from build123d import *

# Parameters (mm, degrees)
SKETCH1_R           = 30
BOSS_EXTRUDE1_DEPTH = 9.1
FILLET1_R           = 1.5
SKETCH2_W           = 47
SKETCH2_H           = 36.6
CUT_EXTRUDE1_DEPTH  = 4.1
SKETCH3_R           = 1.5
CUT_EXTRUDE2_DEPTH  = 43.720018867
CUT_EXTRUDE3_DEPTH  = 3
SKETCH5_R           = 1
CUT_EXTRUDE4_DEPTH  = 43.862687891


with BuildPart() as part:
    # Sketch1 → Boss-Extrude1 (new body)
    with BuildSketch(Plane(origin=(0, 0, 0), x_dir=(1, 0, 0), z_dir=(0, 1, 0))):
        with Locations(Location((0, 0, 0), (0, 0, 270))):
            Circle(SKETCH1_R)
    extrude(amount=BOSS_EXTRUDE1_DEPTH)

    # Fillet1
    fillet1_edges = [part.edges().sort_by_distance(p)[0] for p in [
        (0, 9.1, -30),
    ]]
    fillet(fillet1_edges, radius=FILLET1_R)

    # Sketch2 → Cut-Extrude1 (cut)
    with BuildSketch(Plane(origin=(0, 9.1, 0), x_dir=(1, 0, 0), z_dir=(0, 1, 0))):
        Rectangle(SKETCH2_W, SKETCH2_H)
    extrude(amount=-CUT_EXTRUDE1_DEPTH, mode=Mode.SUBTRACT)

    # Sketch3 → Cut-Extrude2 (cut, through all)
    with BuildSketch(Plane(origin=(0, 5, 0), x_dir=(1, 0, 0), z_dir=(0, 1, 0))):
        with Locations(Location((11.75, 0, 0), (0, 0, 270))):
            Circle(SKETCH3_R)
        with Locations(Location((-11.75, 0, 0), (0, 0, 90))):
            Circle(SKETCH3_R)
    extrude(amount=-CUT_EXTRUDE2_DEPTH, mode=Mode.SUBTRACT)

    # Sketch4 → Cut-Extrude3 (cut)
    with BuildSketch(Plane.XZ):
        with BuildLine():
            Line((-2.389129319, 14.428169014), (-3.73301456, 0.356514085))
            ThreePointArc((-3.73301456, 0.356514085), (-3.75, 0), (-3.73301456, -0.356514085))
            Line((-3.73301456, -0.356514085), (-2.389129319, -14.428169014))
            ThreePointArc((-2.389129319, -14.428169014), (0, -16.6), (2.389129319, -14.428169014))
            Line((2.389129319, -14.428169014), (3.73301456, -0.356514085))
            ThreePointArc((3.73301456, -0.356514085), (3.75, 0), (3.73301456, 0.356514085))
            Line((3.73301456, 0.356514085), (2.389129319, 14.428169014))
            ThreePointArc((2.389129319, 14.428169014), (0, 16.6), (-2.389129319, 14.428169014))
        make_face()
    extrude(amount=-CUT_EXTRUDE3_DEPTH, mode=Mode.SUBTRACT)

    # Sketch5 → Cut-Extrude4 (cut, through all)
    with BuildSketch(Plane.XZ.offset(-3)):
        with Locations(Location((0, 0, 0), (0, 0, 270))):
            Circle(SKETCH5_R)
    extrude(amount=-CUT_EXTRUDE4_DEPTH, mode=Mode.SUBTRACT)


solid = part.part
Model file for the job. Use its own axes, mm. A direction names the side the tool comes from. Give positions to 0.01 mm unless a question says otherwise; leave off trailing zeros. Loops run counter-clockwise (first coordinate to the right, second up) from the corner with the lowest first, then second, coordinate; pieces in that order, holes last. Notation, with made-up numbers: (20, 77.5) -> (49, 77.5) arc R11 cw to (49, 85.5) -> close; hole circle Ø7 at (-8.75, 37). An arc over 180 degrees is marked (long way). Use a Markdown table: item, result. Add a question column.
(1) Wall check: line 1 along X through (y, z) = (2.6, 0); line 2 along X through (y, z) = (3.7, 0); line 3 along Z through (x, y) = (23, 8). Give the ranges that are in metal, low to high.
(2) Tool access for faces 4 (the flat face through (23.5, 7, 0)), 5 (the cylindrical face through (0, 1.5, 16.6)), 6 (the flat face through (-25, 9.1, 0)): list every direction of +Z, -Z, +X, -X, +Y, -Y with a clear straight run to the whole face (end or side of a thin tool).
(3) Slice it at A-A on x = 0. List the corners of the cut face in (y, z), and give its area (3 significant figures).
(4) Slice it at B-B on y = 1.25. List the corners of the cut face in (x, z), and give its area (3 significant figures).
(5) Drop flat-ended pins along their axis: pin 1 Ø1.2 at (x, y) = (-1.5, 7.5) entering from -Z; pin 2 Ø1.5 at (x, z) = (-10.5, 6.5) entering from +Y; pin 3 Ø1.5 at (y, z) = (2, 9.5) entering from +X; pin 4 Ø8.5 at (x, z) = (-1.5, -4) entering from -Y. Give the stop position or say it passes through.
(6) Mould opens along X. For faces 1 (the flat face through (0, 7, -18.3)), 2 (the flat face through (-6, 0, 0)), 3 (the flat face through (2, 3, 0)) say: +X half, -X half, draft (parallel to the pull), parting line (faces both ways), or undercut.
(7) Slice it at C-C on y = 6. List the corners of the cut face in (x, z).
Filled sheet:
| question | item | result |
|---|---|---|
| 1 | line 1 | -30 to -13.25, -10.25 to -3.75, 3.75 to 10.25, 13.25 to 30 |
| 1 | line 2 | -30 to -13.25, -10.25 to -1, 1 to 10.25, 13.25 to 30 |
| 1 | line 3 | -19.18 to -18.3, 18.3 to 19.18 |
| 2 | face 4 | +Y |
| 2 | face 5 | -Y |
| 2 | face 6 | +Z, -Z, +X, -X, +Y |
| 3 | outline | (0, -30) -> (7.6, -30) arc R1.5 ccw to (9.1, -28.5) -> (9.1, -18.3) -> (5, -18.3) -> (5, -1) -> (3, -1) -> (3, -16.6) -> (0, -16.6) -> close; (0, 16.6) -> (3, 16.6) -> (3, 1) -> (5, 1) -> (5, 18.3) -> (9.1, 18.3) -> (9.1, 28.5) arc R1.5 ccw to (7.6, 30) -> (0, 30) -> close |
| 3 | area | 291 mm2 |
| 4 | outline | circle Ø60 at (0, 0); hole circle Ø3 at (-11.75, 0); hole (-3.73, -0.36) -> (-2.39, -14.43) arc R2.4 ccw to (2.39, -14.43) -> (3.73, -0.36) arc R3.75 ccw to (3.73, 0.36) -> (2.39, 14.43) arc R2.4 ccw to (-2.39, 14.43) -> (-3.73, 0.36) arc R3.75 ccw to start; hole circle Ø3 at (11.75, 0) |
| 4 | area | 2,620 mm2 |
| 5 | pin 1 | z = -29.99 |
| 5 | pin 2 | y = 5 |
| 5 | pin 3 | x = 28.7 |
| 5 | pin 4 | y = 0 |
| 6 | face 1 | undercut |
| 6 | face 2 | draft |
| 6 | face 3 | undercut |
| 7 | outline | circle Ø60 at (0, 0); hole (-23.5, -18.3) -> (23.5, -18.3) -> (23.5, 18.3) -> (-23.5, 18.3) -> close |
